Drawing for the job (mm, zero at the part's lowest x, y, z). Coordinates: 2 decimals unless noted, no trailing zeros. Write each loop counter-clockwise with the first axis right and the second up, starting at its lowest first coordinate (ties: lowest second). Pieces come first, ordered by that corner, then holes. Notation, with made-up numbers: M -32.5,49 L 13.5,49 A17 cw 13.5,71 Z; hole C -35.5,-20 d8. An arc over 180 degrees is marked long. Put each result on its own line as item: value. Start each with the question number.
Q1. Drill centre lines: line 1 along X through (y, z) = (0.4, 1.5); line 2 along X through (y, z) = (1.55, 14); line 3 along Z through (x, y) = (4, 1.45). Where is each one in solid material? Low to high.
Q2. Cut at B-B (z = 2.25). Write the cut outline in (x, y), then the cut area to 3 significant figures.
Q3. Cut at A-A (z = 13.5). Write the cut outline in (x, y), then the cut area to 3 significant figures.
Q4. Drop flat-ended pins along their axis: pin 1 (1.5 mm diameter, centred on x = 1, y = 1.5, fed in from +Z); pin 2 (1.5 mm diameter, centred on y = 1, z = 14, fed in from -X); pin 3 (0.9 mm diameter, centred on y = 1.5, z = 1.5, fed in from +X). Give the stop position or say it passes through.
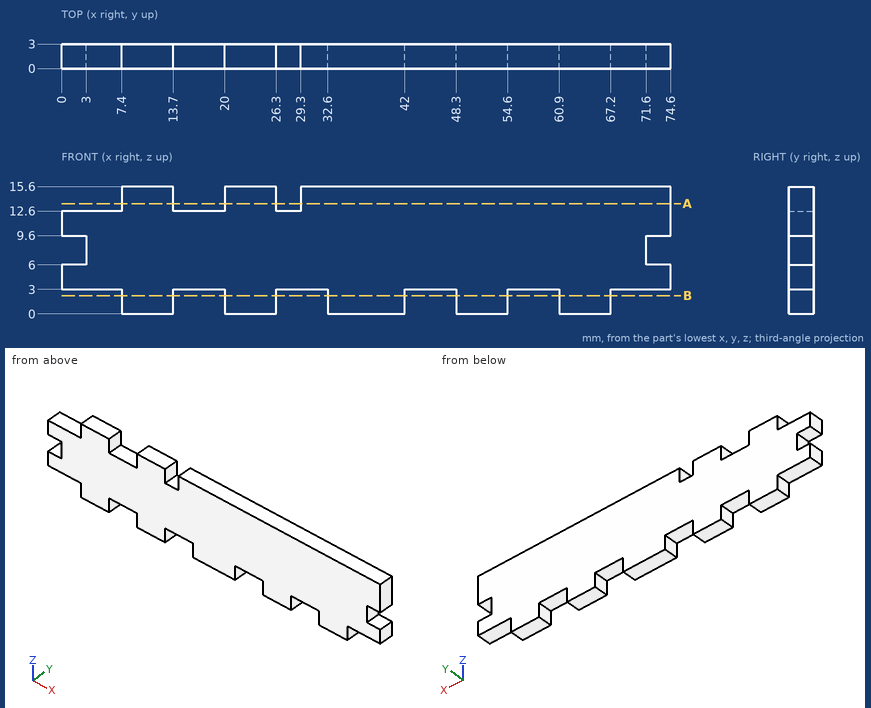
Computed values:
1. line 1: 7.4 to 13.7, 20 to 26.3, 32.6 to 42, 48.3 to 54.6, 60.9 to 67.2
1. line 2: 7.4 to 13.7, 20 to 26.3, 29.3 to 74.6
1. line 3: 3 to 12.6
2. outline: M 7.4,0 L 13.7,0 L 13.7,3 L 7.4,3 Z; M 20,0 L 26.3,0 L 26.3,3 L 20,3 Z; M 32.6,0 L 42,0 L 42,3 L 32.6,3 Z; M 48.3,0 L 54.6,0 L 54.6,3 L 48.3,3 Z; M 60.9,0 L 67.2,0 L 67.2,3 L 60.9,3 Z
2. area: 104 mm2
3. outline: M 7.4,0 L 13.7,0 L 13.7,3 L 7.4,3 Z; M 20,0 L 26.3,0 L 26.3,3 L 20,3 Z; M 29.3,0 L 74.6,0 L 74.6,3 L 29.3,3 Z
3. area: 174 mm2
4. pin 1: z = 12.6
4. pin 2: x = 7.4
4. pin 3: x = 67.2
